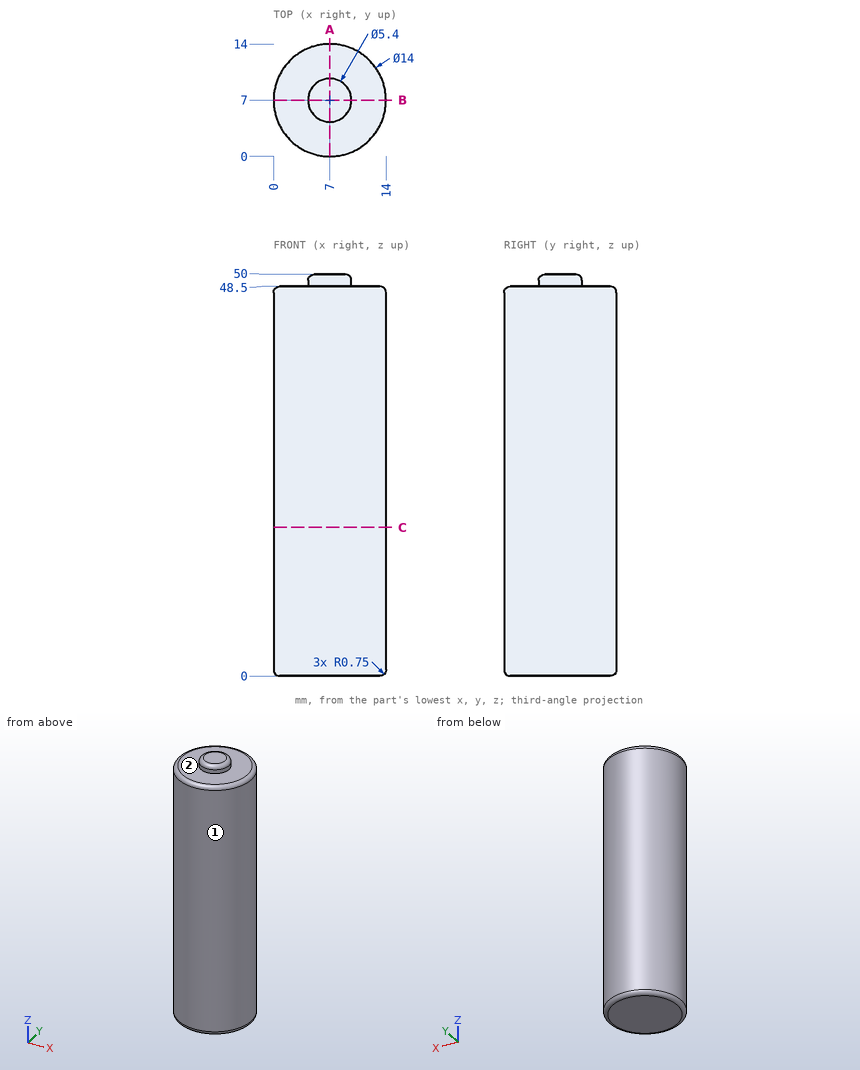
Part print with two shaded views. Sizes in mm from the minimum x, y, z corner. A direction names the side the tool comes from. Give positions to 0.01 mm unless a question says otherwise; leave off trailing zeros. Order: outer loops, then holes, each group sorted by start corner. A loop starts at its lowest first (then second) coordinate and runs counter-clockwise, first axis right, second up.
(1) Flat gauge pins, fed straight in: pin 1 (2 mm diameter, centred on x = 4, z = 13.5, fed in from +Y); pin 2 (4 mm diameter, centred on y = 12, z = 38.5, fed in from -X). Where does each tip first touch, or does it go through?
(2) Tool access for the marked faces 1 and 2: list every direction of +Z, -Z, +X, -X, +Y, -Y with a clear straight run to the whole face (end or side of a thin tool).
(3) Drill centre lines: L1, parallel to Z at x = 3.5, y = 4; L2, parallel to Y at x = 6.75, z = 45; L3, parallel to X at y = 12.75, z = 3. Where is each one in solid material? Low to high.
(4) Saw through at A-A, the plane x = 7. Give the cut face in (y, z), then the cut area to 3 significant figures.
(5) Saw through at C-C, the plane z = 18.5. Give the cut face in (x, y), then the cut area to 3 significant figures.
Results found:
1. pin 1: stops at y = 13.71
1. pin 2: stops at x = 0.68
2. face 1: +Z, -Z
2. face 2: +Z
3. L1: z = 0 to 48.5
3. L2: y = 0 to 14
3. L3: x = 3.01 to 10.99
4. outline: (0, 0.75) arc R0.75 ccw to (0.75, 0) - (13.25, 0) arc R0.75 ccw to (14, 0.75) - (14, 47.75) arc R0.75 ccw to (13.25, 48.5) - (9.7, 48.5) - (9.7, 49.25) arc R0.75 ccw to (8.95, 50) - (5.05, 50) arc R0.75 ccw to (4.3, 49.25) - (4.3, 48.5) - (0.75, 48.5) arc R0.75 ccw to (0, 47.75) - close
4. area: 686 mm2
5. outline: circle Ø14 at (7, 7)
5. area: 154 mm2
